For this review, take the finished solid that the model builds, in its own axes (mm). A direction names the side the tool comes from. Round coordinates to 2 decimals unless told otherwise and drop trailing zeros. Write each loop counter-clockwise with the first axis right and the second up, starting at its lowest first coordinate (ties: lowest second). Pieces come first, ordered by that corner, then holes. Notation, with made-up numbers: (-29, 1.25) -> (-6, 1.25) arc R12 cw to (-6, 17.25) -> close; hole circle Ø5 at (83, 39.5). An arc over 180 degrees is marked (long way). Write each question's results on one line, items separated by ' | '. Start each with the question number.
Item 1: Clearance check with flat-ended pins moving along their axes: pin 1 (3 mm diameter, centred on y = -27, z = 29, fed in from +X); pin 2 (8 mm diameter, centred on x = -27.5, z = 24.5, fed in from +Y); pin 3 (1 mm diameter, centred on x = -25, z = 17.5, fed in from -Y). State where each tip first meets the part, or that it passes through.
Item 2: Add section B-B (z = 17.5). State the section outline as (x, y) points, plus the area to 3 significant figures.
Item 3: To check wall thickness, follow line 1 along X through (y, z) = (-22, 20); line 2 along Z through (x, y) = (28, 17); line 3 along X through (y, z) = (-11, 6.5). State the ranges of each line that lie inside material, in increasing order.
Item 4: Tool access review of faces 4 (the flat face through (7, 7, 2)), 5 (the flat face through (-25, -20, 25)), 6 (the flat face through (-20, 25, 25)): name each direction out of +Z, -Z, +X, -X, +Y, -Y from which nothing blocks a thin tool from reaching the whole face with its end or side.
Item 5: Add section D-D (z = 7). State the section outline as (x, y) points, plus the area to 3 significant figures.
Item 6: The part is to be moulded in two halves that separate along X. For faces 1 (the flat face through (30, -25, 25)), 2 (the flat face through (-25, 20, 25)), 3 (the flat face through (20, 25, 25)), say which applies: +X half, -X half, draft (parallel to the pull), parting line (faces both ways), or undercut.
from build123d import *

# Parameters (mm, degrees)
F0_W     = 80
F0_H     = 80
F1_DEPTH = 10
F2_SIZE2 = 9.99999
F2_SIZE  = 9.99999
F3_W     = 10
F3_H     = 10
F4_DEPTH = 30
F6_DEPTH = 8


# Not quite as in the source:
# - a fillet or chamfer is up to 0.001 mm smaller than in the source, because OpenCascade refuses the exact size


with BuildPart() as f1:
    # F0 (on Top) → F1 (new body)
    with BuildSketch(Plane.XY):
        Rectangle(F0_W, F0_H)
    extrude(amount=F1_DEPTH)

    # F2 (size 10 and 10 in the source; OpenCascade refuses exactly that, so slightly less here)
    f2_edges = [f1.edges().sort_by_distance(p)[0] for p in [
        (0, 40, 10),
        (-40, 0, 10),
        (0, -40, 10),
        (40, 0, 10),
    ]]
    chamfer(f2_edges, length=F2_SIZE, length2=F2_SIZE2)

    # F3 (on face) → F4 (join)
    with BuildSketch(Plane.XY.offset(10)):
        with Locations((-25, 25)):
            Rectangle(F3_W, F3_H)
        with Locations((-25, -25)):
            Rectangle(F3_W, F3_H)
        with Locations((25, 25)):
            Rectangle(F3_W, F3_H)
        with Locations((25, -25)):
            Rectangle(F3_W, F3_H)
    extrude(amount=F4_DEPTH)

    # F5 (on face) → F6 (cut)
    with BuildSketch(Plane.XY.offset(10)):
        with BuildLine():
            Line((-3.8890872965, 3.8890872965), (-10.2530483272, 10.2530483272))
            ThreePointArc((-10.2530483272, 10.2530483272), (-10.2530483272, 3.8890872965), (-3.8890872965, 3.8890872965))
        make_face()
        with BuildLine():
            ThreePointArc((-2.5710678119, 7.0710678119), (-5.3489923662, 11.2285257082), (-10.2530483272, 10.2530483272))
            Line((-10.2530483272, 10.2530483272), (-3.8890872965, 3.8890872965))
            ThreePointArc((-3.8890872965, 3.8890872965), (-2.9136099156, 5.3489923662), (-2.5710678119, 7.0710678119))
        make_face()
        with BuildLine():
            ThreePointArc((10.2530483272, 10.2530483272), (3.8890872965, 10.2530483272), (3.8890872965, 3.8890872965))
            Line((3.8890872965, 3.8890872965), (10.2530483272, 10.2530483272))
        make_face()
        with BuildLine():
            Line((10.2530483272, 10.2530483272), (3.8890872965, 3.8890872965))
            ThreePointArc((3.8890872965, 3.8890872965), (8.7931432575, 2.9136099156), (11.5710678119, 7.0710678119))
            ThreePointArc((11.5710678119, 7.0710678119), (11.2285257082, 8.7931432575), (10.2530483272, 10.2530483272))
        make_face()
        with BuildLine():
            Line((-10.2530483272, -10.2530483272), (-3.8890872965, -3.8890872965))
            ThreePointArc((-3.8890872965, -3.8890872965), (-10.2530483272, -3.8890872965), (-10.2530483272, -10.2530483272))
        make_face()
        with BuildLine():
            ThreePointArc((-2.5710678119, -7.0710678119), (-2.9136099156, -5.3489923662), (-3.8890872965, -3.8890872965))
            Line((-3.8890872965, -3.8890872965), (-10.2530483272, -10.2530483272))
            ThreePointArc((-10.2530483272, -10.2530483272), (-5.3489923662, -11.2285257082), (-2.5710678119, -7.0710678119))
        make_face()
        with BuildLine():
            Line((10.2530483272, -10.2530483272), (3.8890872965, -3.8890872965))
            ThreePointArc((3.8890872965, -3.8890872965), (3.8890872965, -10.2530483272), (10.2530483272, -10.2530483272))
        make_face()
        with BuildLine():
            ThreePointArc((11.5710678119, -7.0710678119), (8.7931432575, -2.9136099156), (3.8890872965, -3.8890872965))
            Line((3.8890872965, -3.8890872965), (10.2530483272, -10.2530483272))
            ThreePointArc((10.2530483272, -10.2530483272), (11.2285257082, -8.7931432575), (11.5710678119, -7.0710678119))
        make_face()
    extrude(amount=-F6_DEPTH, mode=Mode.SUBTRACT)


solid = f1.part
Responses:
1) pin 1: stops at x = 30 | pin 2: stops at y = 30 | pin 3: stops at y = -30
2) outline: (-30, -30) -> (-20, -30) -> (-20, -20) -> (-30, -20) -> close; (-30, 20) -> (-20, 20) -> (-20, 30) -> (-30, 30) -> close; (20, -30) -> (30, -30) -> (30, -20) -> (20, -20) -> close; (20, 20) -> (30, 20) -> (30, 30) -> (20, 30) -> close | area: 400 mm^2
3) line 1: x = -30 to -20, 20 to 30 | line 2: z = 0 to 10 | line 3: x = -33.5 to -9.27, -4.88 to 4.88, 9.27 to 33.5
4) face 4: +Z | face 5: +Z, +X, -X | face 6: +Z, +Y, -Y
5) outline: (-33, -33) -> (33, -33) -> (33, 33) -> (-33, 33) -> close; hole circle Ø9 at (-7.07, -7.07); hole circle Ø9 at (-7.07, 7.07); hole circle Ø9 at (7.07, -7.07); hole circle Ø9 at (7.07, 7.07) | area: 4,100 mm^2
6) face 1: +X half | face 2: draft | face 3: undercut
